Answer from the drawing. Dimensions are ordinates in mm from the lowest x, y and z of the part. A direction names the side the tool comes from. Round coordinates to 2 decimals unless told otherwise and drop trailing zeros. Loops run counter-clockwise (first coordinate to the right, second up) from the corner with the lowest first, then second, coordinate; pieces in that order, holes last. Notation, with made-up numbers: (53, -37) -> (69, -37) arc R17 ccw to (69, -10) -> close; hole circle Ø6 at (-15.5, 67.5). An arc over 180 degrees is marked (long way). One line per question, with ' | ' between items.
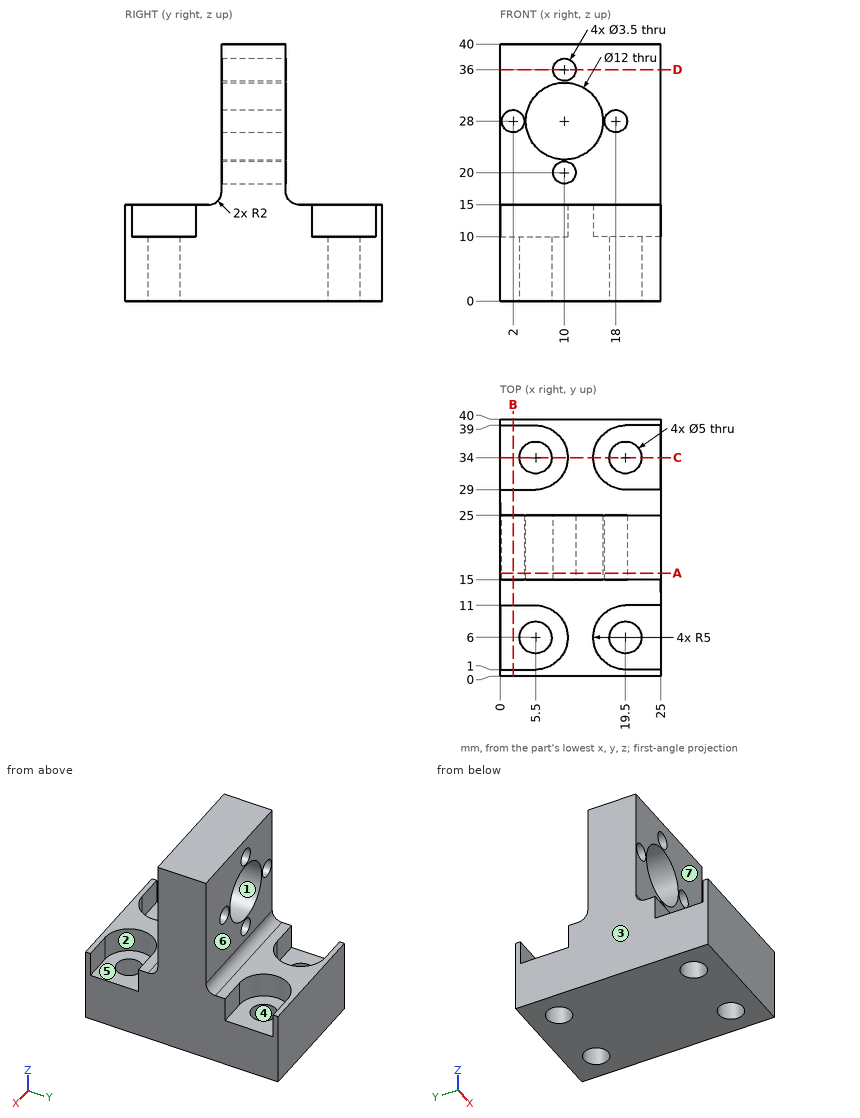
Q1. Given pin 1 Ø12 at (x, y) = (5, 26) entering from +Z; pin 2 Ø11 at (x, y) = (7, 35) entering from +Z; pin 3 Ø6 at (x, y) = (5.5, 6) entering from +Z; pin 4 Ø14.5 at (x, y) = (6.5, 6.5) entering from +Z, each flat-ended and moving along its own axis, determine where each tip first touches the part or whether it passes through.
Numbers:
pin 1: z = 40 | pin 2: z = 15 | pin 3: z = 10 | pin 4: z = 15.15
Q2. For a pull along X with two mould halves and no side action, classify the marked faces 1, 2, 3 and 4 as pulls with the +X half, pulls with the -X half, needs draft (parallel to the pull), parting line crosses it, or undercut.
Numbers:
face 1: undercut | face 2: pulls with the +X half | face 3: pulls with the -X half | face 4: undercut
Q3. A cutting plane is placed at D-D on z = 36. Give the vertices of the cut face in (x, y).
Numbers:
outline: (0, 15) -> (8.25, 15) -> (8.25, 25) -> (0, 25) -> close; (11.75, 15) -> (25, 15) -> (25, 25) -> (11.75, 25) -> close
Q4. A cutting plane is placed at B-B on x = 2. Give the vertices of the cut face in (y, z), plus the area to 3 significant figures.
Numbers:
outline: (0, 0) -> (40, 0) -> (40, 15) -> (39, 15) -> (39, 10) -> (29, 10) -> (29, 15) -> (27, 15) arc R2 cw to (25, 17) -> (25, 26.25) -> (15, 26.25) -> (15, 17) arc R2 cw to (13, 15) -> (11, 15) -> (11, 10) -> (1, 10) -> (1, 15) -> (0, 15) -> close; (15, 29.75) -> (25, 29.75) -> (25, 40) -> (15, 40) -> close | area: 717 mm^2
Q5. A cutting plane is placed at A-A on y = 16. Give the vertices of the cut face in (x, z), plus the area to 3 significant figures.
Numbers:
outline: (0, 0) -> (25, 0) -> (25, 40) -> (0, 40) -> close; hole circle Ø3.5 at (2, 28); hole circle Ø12 at (10, 28); hole circle Ø3.5 at (10, 20); hole circle Ø3.5 at (10, 36); hole circle Ø3.5 at (18, 28) | area: 848 mm^2
Q6. Find the intervals of material crossed by line 1 (Y direction, x = 5.5, z = 3); line 2 (X direction, y = 19.75, z = 28); line 3 (X direction, y = 6, z = 6), in increasing order. Write a range as from..to.
Numbers:
line 1: 0..3.5, 8.5..31.5, 36.5..40 | line 2: 0..0.25, 3.75..4, 16..16.25, 19.75..25 | line 3: 0..3, 8..17, 22..25
Q7. For the marked faces 5, 6 and 7, determine the directions among +Z, -Z, +X, -X, +Y, -Y from which every point of the face is accessible in a straight line to the end or side of a thin tool.
Numbers:
face 5: +Z, +X | face 6: +Z, +X, -X, +Y | face 7: +Z, +X, -X, -Y
Q8. A cutting plane is placed at C-C on y = 34. Give the vertices of the cut face in (x, z), plus the area to 3 significant figures.
Numbers:
outline: (0, 0) -> (3, 0) -> (3, 10) -> (0, 10) -> close; (8, 0) -> (17, 0) -> (17, 10) -> (14.5, 10) -> (14.5, 15) -> (10.5, 15) -> (10.5, 10) -> (8, 10) -> close; (22, 0) -> (25, 0) -> (25, 10) -> (22, 10) -> close | area: 170 mm^2
